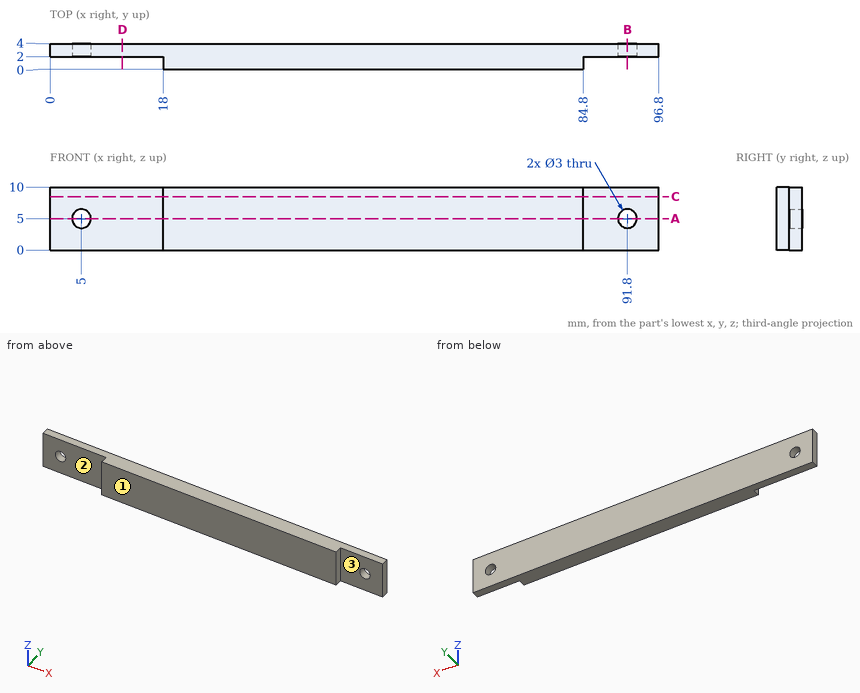
Input: dimensioned drawing with shaded views. Units: mm. Origin: part minimum x, y, z. A direction names the side the tool comes from. Give positions to 0.01 mm unless a question says otherwise; leave off trailing zeros. Write each loop counter-clockwise with the first axis right and the second up, starting at its lowest first coordinate (ties: lowest second). Pieces come first, ordered by that corner, then holes. Notation, with made-up numbers: (5.25, -9) -> (21.25, -9) arc R13 ccw to (21.25, 5) -> close; hole circle Ø8 at (42, 31.5). An arc over 180 degrees is marked (long way). Return JSON: item names as keys, results as strings. Group by question number.
1. Section A-A, the plane z = 5. Output: boundary loops of the cut face in (x, y), then the cut area to 3 significant figures.
2. Material intervals for line 1 (X direction, y = 3.55, z = 5); line 2 (X direction, y = 3.4, z = 6); line 3 (Y direction, x = 90.5, z = 3.25), sorted ascending. Write a range as from..to.
3. Section C-C, the plane z = 8.5. Output: boundary loops of the cut face in (x, y).
4. Pin query (flat end, axial travel): pin 1 Ø1.8 at (x, z) = (5, 5) entering from -Y; pin 2 Ø5 at (x, z) = (9.5, 5) entering from -Y; pin 3 Ø2 at (y, z) = (0.5, 5.5) entering from -X. Return the tip coordinate at first contact, or that it passes through.
5. Section D-D, the plane x = 11.5. Output: boundary loops of the cut face in (y, z).
6. Access query for the marked faces 1, 2 and 3. Directions: +Z, -Z, +X, -X, +Y, -Y. A direction counts if a zero-diameter tool reaches every point of the face in a straight line with its end or side. Return the directions, or none.
7. Section B-B, the plane x = 91.8. Output: boundary loops of the cut face in (y, z).
Determined:
{
 "1": {"outline": "(0, 2) -> (3.5, 2) -> (3.5, 4) -> (0, 4) -> close; (6.5, 2) -> (18, 2) -> (18, 0) -> (84.8, 0) -> (84.8, 2) -> (90.3, 2) -> (90.3, 4) -> (6.5, 4) -> close; (93.3, 2) -> (96.8, 2) -> (96.8, 4) -> (93.3, 4) -> close", "area": "315 mm2"},
 "2": {"line 1": "x = 0..3.5, 6.5..90.3, 93.3..96.8", "line 2": "x = 0..3.88, 6.12..90.68, 92.92..96.8", "line 3": "y = 2..4"},
 "3": {"outline": "(0, 2) -> (18, 2) -> (18, 0) -> (84.8, 0) -> (84.8, 2) -> (96.8, 2) -> (96.8, 4) -> (0, 4) -> close"},
 "4": {"pin 1": "passes through", "pin 2": "stops at y = 2", "pin 3": "stops at x = 18"},
 "5": {"outline": "(2, 0) -> (4, 0) -> (4, 10) -> (2, 10) -> close"},
 "6": {"face 1": "+Z, -Z, +X, -X, -Y", "face 2": "+Z, -Z, -X, -Y", "face 3": "+Z, -Z, +X, -Y"},
 "7": {"outline": "(2, 0) -> (4, 0) -> (4, 3.5) -> (2, 3.5) -> close; (2, 6.5) -> (4, 6.5) -> (4, 10) -> (2, 10) -> close"}
}
